from build123d import *

# Parameters (mm, degrees)
BOSS_EXTRUDE1_DEPTH = 5
SKETCH2_R           = 5
CUT_EXTRUDE1_DEPTH  = 153.47950682
SKETCH5_R           = 2.5
CUT_EXTRUDE4_DEPTH  = 12.5
CUT_EXTRUDE5_DEPTH  = 10
SKETCH7_R           = 2.5
CUT_EXTRUDE6_DEPTH  = 10
SKETCH8_R           = 2.5
CUT_EXTRUDE7_DEPTH  = 10
SKETCH9_R           = 8.75
CUT_EXTRUDE8_DEPTH  = 2.5


with BuildPart() as part:
    # Sketch1 → Boss-Extrude1 (new body)
    with BuildSketch(Plane.XY):
        with BuildLine():
            ThreePointArc((95.335601491, -10.870848257), (100, 0), (95.335601491, 10.870848257))
            ThreePointArc((95.335601491, 10.870848257), (66.361018737, 51.737458432), (54.990773904, 100.526020671))
            ThreePointArc((54.990773904, 100.526020671), (47.847440062, 112.783492655), (33.684210526, 113.60554311))
            ThreePointArc((33.684210526, 113.60554311), (0, 106.168439698), (-33.684210526, 113.60554311))
            ThreePointArc((-33.684210526, 113.60554311), (-47.847440062, 112.783492655), (-54.990773904, 100.526020671))
            ThreePointArc((-54.990773904, 100.526020671), (-66.361018737, 51.737458432), (-95.335601491, 10.870848257))
            ThreePointArc((-95.335601491, 10.870848257), (-100, 0), (-95.335601491, -10.870848257))
            ThreePointArc((-95.335601491, -10.870848257), (-66.361018737, -51.737458432), (-54.990773904, -100.526020671))
            ThreePointArc((-54.990773904, -100.526020671), (-47.847440062, -112.783492655), (-33.684210526, -113.60554311))
            ThreePointArc((-33.684210526, -113.60554311), (0, -106.168439698), (33.684210526, -113.60554311))
            ThreePointArc((33.684210526, -113.60554311), (47.847440062, -112.783492655), (54.990773904, -100.526020671))
            ThreePointArc((54.990773904, -100.526020671), (66.361018737, -51.737458432), (95.335601491, -10.870848257))
        make_face()
    extrude(amount=BOSS_EXTRUDE1_DEPTH)

    # Sketch2 → Cut-Extrude1 (cut, through all)
    with BuildSketch(Plane(origin=(0, 0, 0), x_dir=(-1, 0, 0), z_dir=(0, 0, -1))):
        with Locations((-40, 100)):
            Circle(SKETCH2_R)
        with Locations((-85, 0)):
            Circle(SKETCH2_R)
        with Locations(Location((85, 0, 0), (0, 0, 180))):
            Circle(SKETCH2_R)
        with Locations(Location((40, 100, 0), (0, 0, 180))):
            Circle(SKETCH2_R)
        with Locations((40, -100)):
            Circle(SKETCH2_R)
        with Locations(Location((-40, -100, 0), (0, 0, 180))):
            Circle(SKETCH2_R)
    extrude(amount=-CUT_EXTRUDE1_DEPTH, mode=Mode.SUBTRACT)

    # Sketch5 → Cut-Extrude4 (cut)
    with BuildSketch(Plane(origin=(0, 0, 0), x_dir=(-1, 0, 0), z_dir=(0, 0, -1))):
        with Locations((20, 95)):
            Circle(SKETCH5_R)
        with Locations((0, 95)):
            Circle(SKETCH5_R)
        with Locations((10, 95)):
            Circle(SKETCH5_R)
        with Locations(Location((10, -95, 0), (0, 0, 180))):
            Circle(SKETCH5_R)
        with Locations(Location((0, -95, 0), (0, 0, 180))):
            Circle(SKETCH5_R)
        with Locations(Location((20, -95, 0), (0, 0, 180))):
            Circle(SKETCH5_R)
        with Locations(Location((-20, 95, 0), (0, 0, 180))):
            Circle(SKETCH5_R)
        with Locations(Location((-10, 95, 0), (0, 0, 180))):
            Circle(SKETCH5_R)
        with Locations((-20, -95)):
            Circle(SKETCH5_R)
        with Locations((-10, -95)):
            Circle(SKETCH5_R)
    extrude(amount=-CUT_EXTRUDE4_DEPTH, mode=Mode.SUBTRACT)

    # Sketch6 → Cut-Extrude5 (cut)
    with BuildSketch(Plane.XY.offset(5)):
        with BuildLine():
            Line((42.5, 75), (42.5, 45))
            ThreePointArc((42.5, 45), (40, 42.5), (37.5, 45))
            Line((37.5, 45), (37.5, 75))
            ThreePointArc((37.5, 75), (40, 77.5), (42.5, 75))
        make_face()
        with BuildLine():
            Line((22.5, 75), (22.5, 45))
            ThreePointArc((22.5, 45), (20, 42.5), (17.5, 45))
            Line((17.5, 45), (17.5, 75))
            ThreePointArc((17.5, 75), (20, 77.5), (22.5, 75))
        make_face()
        with BuildLine():
            Line((2.5, 75), (2.5, 45))
            ThreePointArc((2.5, 45), (0, 42.5), (-2.5, 45))
            Line((-2.5, 45), (-2.5, 75))
            ThreePointArc((-2.5, 75), (0, 77.5), (2.5, 75))
        make_face()
        with BuildLine():
            Line((-17.5, 75), (-17.5, 45))
            ThreePointArc((-17.5, 45), (-20, 42.5), (-22.5, 45))
            Line((-22.5, 45), (-22.5, 75))
            ThreePointArc((-22.5, 75), (-20, 77.5), (-17.5, 75))
        make_face()
        with BuildLine():
            Line((-37.5, 75), (-37.5, 45))
            ThreePointArc((-37.5, 45), (-40, 42.5), (-42.5, 45))
            Line((-42.5, 45), (-42.5, 75))
            ThreePointArc((-42.5, 75), (-40, 77.5), (-37.5, 75))
        make_face()
        with BuildLine():
            Line((42.5, 15), (42.5, -15))
            ThreePointArc((42.5, -15), (40, -17.5), (37.5, -15))
            Line((37.5, -15), (37.5, 15))
            ThreePointArc((37.5, 15), (40, 17.5), (42.5, 15))
        make_face()
        with BuildLine():
            Line((22.5, 15), (22.5, -15))
            ThreePointArc((22.5, -15), (20, -17.5), (17.5, -15))
            Line((17.5, -15), (17.5, 15))
            ThreePointArc((17.5, 15), (20, 17.5), (22.5, 15))
        make_face()
        with BuildLine():
            Line((2.5, 15), (2.5, -15))
            ThreePointArc((2.5, -15), (0, -17.5), (-2.5, -15))
            Line((-2.5, -15), (-2.5, 15))
            ThreePointArc((-2.5, 15), (0, 17.5), (2.5, 15))
        make_face()
        with BuildLine():
            Line((-17.5, 15), (-17.5, -15))
            ThreePointArc((-17.5, -15), (-20, -17.5), (-22.5, -15))
            Line((-22.5, -15), (-22.5, 15))
            ThreePointArc((-22.5, 15), (-20, 17.5), (-17.5, 15))
        make_face()
        with BuildLine():
            Line((-37.5, 15), (-37.5, -15))
            ThreePointArc((-37.5, -15), (-40, -17.5), (-42.5, -15))
            Line((-42.5, -15), (-42.5, 15))
            ThreePointArc((-42.5, 15), (-40, 17.5), (-37.5, 15))
        make_face()
        with BuildLine():
            Line((42.5, -45), (42.5, -75))
            ThreePointArc((42.5, -75), (40, -77.5), (37.5, -75))
            Line((37.5, -75), (37.5, -45))
            ThreePointArc((37.5, -45), (40, -42.5), (42.5, -45))
        make_face()
        with BuildLine():
            Line((22.5, -45), (22.5, -75))
            ThreePointArc((22.5, -75), (20, -77.5), (17.5, -75))
            Line((17.5, -75), (17.5, -45))
            ThreePointArc((17.5, -45), (20, -42.5), (22.5, -45))
        make_face()
        with BuildLine():
            Line((2.5, -45), (2.5, -75))
            ThreePointArc((2.5, -75), (0, -77.5), (-2.5, -75))
            Line((-2.5, -75), (-2.5, -45))
            ThreePointArc((-2.5, -45), (0, -42.5), (2.5, -45))
        make_face()
        with BuildLine():
            Line((-17.5, -45), (-17.5, -75))
            ThreePointArc((-17.5, -75), (-20, -77.5), (-22.5, -75))
            Line((-22.5, -75), (-22.5, -45))
            ThreePointArc((-22.5, -45), (-20, -42.5), (-17.5, -45))
        make_face()
        with BuildLine():
            Line((-37.5, -45), (-37.5, -75))
            ThreePointArc((-37.5, -75), (-40, -77.5), (-42.5, -75))
            Line((-42.5, -75), (-42.5, -45))
            ThreePointArc((-42.5, -45), (-40, -42.5), (-37.5, -45))
        make_face()
    extrude(amount=-CUT_EXTRUDE5_DEPTH, mode=Mode.SUBTRACT)

    # Sketch7 → Cut-Extrude6 (cut)
    with BuildSketch(Plane.XY.offset(5)):
        with Locations((-65, 30)):
            Circle(SKETCH7_R)
        with Locations((-55, 30)):
            Circle(SKETCH7_R)
        with Locations((-45, 30)):
            Circle(SKETCH7_R)
        with Locations((-35, 30)):
            Circle(SKETCH7_R)
        with Locations((-25, 30)):
            Circle(SKETCH7_R)
        with Locations((-15, 30)):
            Circle(SKETCH7_R)
        with Locations((-5, 30)):
            Circle(SKETCH7_R)
        with Locations((5, 30)):
            Circle(SKETCH7_R)
        with Locations((15, 30)):
            Circle(SKETCH7_R)
        with Locations((25, 30)):
            Circle(SKETCH7_R)
        with Locations((35, 30)):
            Circle(SKETCH7_R)
        with Locations((45, 30)):
            Circle(SKETCH7_R)
        with Locations((55, 30)):
            Circle(SKETCH7_R)
        with Locations((65, 30)):
            Circle(SKETCH7_R)
        with Locations((65, -30)):
            Circle(SKETCH7_R)
        with Locations((55, -30)):
            Circle(SKETCH7_R)
        with Locations((45, -30)):
            Circle(SKETCH7_R)
        with Locations((35, -30)):
            Circle(SKETCH7_R)
        with Locations((25, -30)):
            Circle(SKETCH7_R)
        with Locations((15, -30)):
            Circle(SKETCH7_R)
        with Locations((5, -30)):
            Circle(SKETCH7_R)
        with Locations((-5, -30)):
            Circle(SKETCH7_R)
        with Locations((-15, -30)):
            Circle(SKETCH7_R)
        with Locations((-25, -30)):
            Circle(SKETCH7_R)
        with Locations((-35, -30)):
            Circle(SKETCH7_R)
        with Locations((-45, -30)):
            Circle(SKETCH7_R)
        with Locations((-55, -30)):
            Circle(SKETCH7_R)
        with Locations((-65, -30)):
            Circle(SKETCH7_R)
    extrude(amount=-CUT_EXTRUDE6_DEPTH, mode=Mode.SUBTRACT)

    # Sketch8 → Cut-Extrude7 (cut)
    with BuildSketch(Plane.XY.offset(5)):
        with Locations((-65, 0)):
            Circle(SKETCH8_R)
        with Locations((-65, 15)):
            Circle(SKETCH8_R)
        with Locations((-65, -15)):
            Circle(SKETCH8_R)
        with Locations((65, -15)):
            Circle(SKETCH8_R)
        with Locations((65, 0)):
            Circle(SKETCH8_R)
        with Locations((65, 15)):
            Circle(SKETCH8_R)
    extrude(amount=-CUT_EXTRUDE7_DEPTH, mode=Mode.SUBTRACT)

    # Sketch9 → Cut-Extrude8 (cut)
    with BuildSketch(Plane(origin=(0, 0, 0), x_dir=(-1, 0, 0), z_dir=(0, 0, -1))):
        with Locations((85, 0)):
            Circle(SKETCH9_R)
        with Locations((40, 100)):
            Circle(SKETCH9_R)
        with Locations((40, -100)):
            Circle(SKETCH9_R)
        with Locations((-40, -100)):
            Circle(SKETCH9_R)
        with Locations((-85, 0)):
            Circle(SKETCH9_R)
        with Locations((-40, 100)):
            Circle(SKETCH9_R)
    extrude(amount=-CUT_EXTRUDE8_DEPTH, mode=Mode.SUBTRACT)


solid = part.part
The model under review builds one solid part; all positions refer to its coordinate system, in mm. A direction names the side the tool comes from. Round coordinates to 2 decimals unless told otherwise and drop trailing zeros. Loops run counter-clockwise (first coordinate to the right, second up) from the corner with the lowest first, then second, coordinate; pieces in that order, holes last. Notation, with made-up numbers: (9, -35.5) - (22, -35.5) arc R22 cw to (22, -26.5) - close; hole circle Ø5 at (31.5, -17). An arc over 180 degrees is marked (long way). Use CSV: the item, a comma, the result in double quotes.
(1) For line 1 (Y direction, x = -40, z = 1.4); line 2 (X direction, y = -102, z = 3.7); line 3 (Y direction, x = -40, z = 4.45), list the stretches that pass through material, from the lowest coordinate up.
Working result:
line 1,"y = -115 to -108.75, -91.25 to -77.5, -42.5 to -17.5, 17.5 to 42.5, 77.5 to 91.25, 108.75 to 115"
line 2,"x = -54.87 to -44.58, -35.42 to 35.42, 44.58 to 54.87"
line 3,"y = -115 to -105, -95 to -77.5, -42.5 to -17.5, 17.5 to 42.5, 77.5 to 95, 105 to 115"
(2) Take a section at B-B, the plane x = -65. Give the boundary of the cut face in (y, z), plus the area to 3 significant figures.
Working result:
outline,"(-54.87, 0) - (-32.5, 0) - (-32.5, 5) - (-54.87, 5) - close; (-27.5, 0) - (-17.5, 0) - (-17.5, 5) - (-27.5, 5) - close; (-12.5, 0) - (-2.5, 0) - (-2.5, 5) - (-12.5, 5) - close; (2.5, 0) - (12.5, 0) - (12.5, 5) - (2.5, 5) - close; (17.5, 0) - (27.5, 0) - (27.5, 5) - (17.5, 5) - close; (32.5, 0) - (54.87, 0) - (54.87, 5) - (32.5, 5) - close"
area,"424 mm^2"
(3) Machinability: for faces 1 (the cylindrical face through (-100, 0, 2)), 2 (the cylindrical face through (-19.9, -17.5, 2.5)), 3 (the flat face through (81, -4, 2.5)), which of the approach directions +Z, -Z, +X, -X, +Y, -Y give a long, thin tool a straight path to every point of the face, cutting with its end or side? Answer none if there is none.
Working result:
face 1,"+Z, -Z, -X"
face 2,"+Z, -Z"
face 3,"-Z"
(4) The part is to be moulded in two halves that separate along X. For faces 4 (the cylindrical face through (56.34, 32.11, 2.54)), 5 (the cylindrical face through (-66.652, -51.095, 2.465)), say which applies: pulls with the +X half, pulls with the -X half, needs draft (parallel to the pull), parting line crosses it, or undercut.
Working result:
face 4,"undercut"
face 5,"pulls with the -X half"
(5) Clearance check with flat-ended pins moving along their axes: P1, Ø8, axis at x = 0, y = 95, coming from the +Z side; P2, Ø9, axis at x = 37, y = -99.5, coming from the -Z side; P3, Ø1.5, axis at x = -31, z = 1, coming from the -Y side; P4, Ø2.5, axis at y = -65.5, z = 3.5, coming from the +X side. State where each tip first meets the part, or that it passes through.
Working result:
P1,"stops at z = 5"
P2,"stops at z = 2.5"
P3,"stops at y = -112.74"
P4,"stops at x = 61.49"
(6) Take a section at D-D, the plane x = 15. Give the boundary of the cut face in (y, z).
Working result:
outline,"(-107.59, 0) - (-32.5, 0) - (-32.5, 5) - (-107.59, 5) - close; (-27.5, 0) - (27.5, 0) - (27.5, 5) - (-27.5, 5) - close; (32.5, 0) - (107.59, 0) - (107.59, 5) - (32.5, 5) - close"
(7) Take a section at C-C, the plane y = -55. Give the boundary of the cut face in (x, z).
Working result:
outline,"(-64.95, 0) - (-42.5, 0) - (-42.5, 5) - (-64.95, 5) - close; (-37.5, 0) - (-22.5, 0) - (-22.5, 5) - (-37.5, 5) - close; (-17.5, 0) - (-2.5, 0) - (-2.5, 5) - (-17.5, 5) - close; (2.5, 0) - (17.5, 0) - (17.5, 5) - (2.5, 5) - close; (22.5, 0) - (37.5, 0) - (37.5, 5) - (22.5, 5) - close; (42.5, 0) - (64.95, 0) - (64.95, 5) - (42.5, 5) - close"
(8) Take a section at A-A, the plane x = -10. Give the boundary of the cut face in (y, z), plus the area to 3 significant figures.
Working result:
outline,"(-106.8, 0) - (-97.5, 0) - (-97.5, 5) - (-106.8, 5) - close; (-92.5, 0) - (92.5, 0) - (92.5, 5) - (-92.5, 5) - close; (97.5, 0) - (106.8, 0) - (106.8, 5) - (97.5, 5) - close"
area,"1,020 mm^2"
